Verification items for the finished model (mm, model axes). A direction names the side the tool comes from. Round coordinates to 2 decimals unless told otherwise and drop trailing zeros. Write each loop counter-clockwise with the first axis right and the second up, starting at its lowest first coordinate (ties: lowest second). Pieces come first, ordered by that corner, then holes. Notation, with made-up numbers: (59, 68.25) - (68, 68.25) arc R22 cw to (68, 86.25) - close; hole circle Ø9 at (-11.5, 47.25). An arc over 180 degrees is marked (long way). Write each question's results on one line, items separated by ' | '.
```python
from build123d import *

# Parameters (mm, degrees)
SKETCH1_R           = 1.651
BOSS_EXTRUDE1_DEPTH = 4.445
SKETCH2_R           = 1.00584
CUT_EXTRUDE1_DEPTH  = 6.973853634


with BuildPart() as part:
    # Sketch1 → Boss-Extrude1 (new body)
    with BuildSketch(Plane.XY):
        Circle(SKETCH1_R)
        Polygon((-0.22225, 2.8575), (0.22225, 2.8575), (0.43815, 1.591799478), (-0.43815, 1.591799478), align=None)
        Polygon((1.859400385, 2.181130789), (1.290107054, 1.030254721), (0.581165462, 1.545330937), (1.499792331, 2.442401334), align=None)
        Polygon((2.786323022, 0.671643751), (1.649287062, 0.075187678), (1.37849547, 0.908598503), (2.648964968, 1.094388372), align=None)
        Polygon((2.648964968, -1.094388372), (1.37849547, -0.908598503), (1.649287062, -0.075187678), (2.786323022, -0.671643751), align=None)
        Polygon((1.499792331, -2.442401334), (0.581165462, -1.545330937), (1.290107054, -1.030254721), (1.859400385, -2.181130789), align=None)
        Polygon((-0.22225, -2.8575), (-0.43815, -1.591799478), (0.43815, -1.591799478), (0.22225, -2.8575), align=None)
        Polygon((-1.859400385, -2.181130789), (-1.290107054, -1.030254721), (-0.581165462, -1.545330937), (-1.499792331, -2.442401334), align=None)
        Polygon((-2.786323022, -0.671643751), (-1.649287062, -0.075187678), (-1.37849547, -0.908598503), (-2.648964968, -1.094388372), align=None)
        Polygon((-2.648964968, 1.094388372), (-1.37849547, 0.908598503), (-1.649287062, 0.075187678), (-2.786323022, 0.671643751), align=None)
        Polygon((-1.499792331, 2.442401334), (-0.581165462, 1.545330937), (-1.290107054, 1.030254721), (-1.859400385, 2.181130789), align=None)
    extrude(amount=BOSS_EXTRUDE1_DEPTH)

    # Sketch2 → Cut-Extrude1 (cut, through all)
    with BuildSketch(Plane.XY.offset(4.445)):
        Circle(SKETCH2_R)
    extrude(amount=-CUT_EXTRUDE1_DEPTH, mode=Mode.SUBTRACT)


solid = part.part
```
(1) Section check A-A (y = 0). Record the cut outline in (x, z) (3 decimals), plus the area to 3 significant figures.
Answer:
outline: (-1.651, 0) - (-1.006, 0) - (-1.006, 4.445) - (-1.651, 4.445) - close; (1.006, 0) - (1.651, 0) - (1.651, 4.445) - (1.006, 4.445) - close | area: 5.74 mm2
(2) Section check B-B (x = -2.3). Record the cut outline in (y, z) (3 decimals).
Answer:
outline: (-1.043, 0) - (-0.417, 0) - (-0.417, 4.445) - (-1.043, 4.445) - close; (0.417, 0) - (1.043, 0) - (1.043, 4.445) - (0.417, 4.445) - close
(3) Thickness scan on L1, parallel to Y at x = 0, z = 3.2; L2, parallel to X at y = -1.65, z = 4; L3, parallel to X at y = -2.05, z = 3.65. Record the ranges inside material, lowest first.
Answer:
L1: -2.86 to -1.01, 1.01 to 2.86 | L2: -1.6 to -0.69, -0.43 to 0.43, 0.69 to 1.6 | L3: -1.79 to -1.1, -0.36 to 0.36, 1.1 to 1.79
(4) Set-up check for faces 5 (the flat face through (-2, 1, 2)), 6 (the flat face through (2.23, 0.38, 2.19)), 7 (the flat face through (-0.33, -2.23, 2.19)), 8 (the flat face through (-1.047, 2, 2.191)): record each of +Z, -Z, +X, -X, +Y, -Y from which the full face is reachable in a straight line by a thin tool's end or side.
Answer:
face 5: +Z, -Z | face 6: +Z, -Z, +X | face 7: +Z, -Z, -Y | face 8: +Z, -Z, +Y
(5) Go/stop test with a flat-tipped pin: pin 1 Ø1.5 at (y, z) = (1.5, 2) entering from +X. Record where the tip stops, or that it passes through.
Answer:
pin 1: x = 2.76
(6) Mould release check, pull along X, two halves, no side actions. Record for faces 1 (the flat face through (-2.21, 0.37, 2.19)), 2 (the flat face through (0.33, 2.23, 2.19)), 3 (the cylindrical face through (-0.8, -0.61, 2.25)), 4 (the flat face through (1.2, 0, 4.445)): released by +X, released by -X, zero draft, split by the parting line, or undercut.
Answer:
face 1: released by -X | face 2: undercut | face 3: undercut | face 4: zero draft
(7) Section check C-C (y = -2). Record the cut outline in (x, z) (3 decimals), plus the area to 3 significant figures.
Answer:
outline: (-1.77, 0) - (-1.047, 0) - (-1.047, 4.445) - (-1.77, 4.445) - close; (-0.369, 0) - (0.369, 0) - (0.369, 4.445) - (-0.369, 4.445) - close; (1.047, 0) - (1.77, 0) - (1.77, 4.445) - (1.047, 4.445) - close | area: 9.70 mm2
(8) Section check D-D (y = -1.35). Record the cut outline in (x, z) (3 decimals).
Answer:
outline: (-1.448, 0) - (1.448, 0) - (1.448, 4.445) - (-1.448, 4.445) - close
